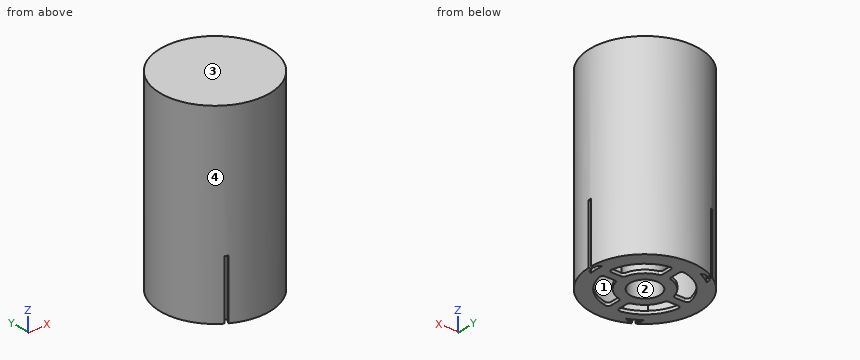
```python
from build123d import *

# Parameters (mm, degrees)
SKETCH_1_R          = 55
EXTRUDE_1_DEPTH     = 190
SKETCH_2_R          = 51.8
CUT_EXTRUDE_1_DEPTH = 186.8
SKETCH_3_R          = 15
CUT_EXTRUDE_2_DEPTH = 10
SKETCH_4_R          = 18.2
SKETCH_4_R_2        = 15
EXTRUDE_2_DEPTH     = 188
SKETCH_5_R          = 55
EXTRUDE_5_DEPTH     = 3.2
EXTRUDE_6_DEPTH     = 1.5
EXTRUDE_START       = -63.2
EXTRUDE_7_DEPTH     = 63.2
CUT_EXTRUDE_START   = -60
CUT_EXTRUDE_4_DEPTH = 60
SKETCH_12_R         = 138.367390037
SKETCH_12_R_2       = 55
CUT_EXTRUDE_5_DEPTH = 135
CUT_EXTRUDE_6_DEPTH = 10


with BuildPart() as part:
    # 草图1 → 凸台-拉伸1 (new body)
    with BuildSketch(Plane.XY):
        Circle(SKETCH_1_R)
    extrude(amount=EXTRUDE_1_DEPTH)

    # 草图2 → 切除-拉伸1 (cut)
    with BuildSketch(Plane.XY.offset(190)):
        Circle(SKETCH_2_R)
    extrude(amount=-CUT_EXTRUDE_1_DEPTH, mode=Mode.SUBTRACT)

    # 草图3 → 切除-拉伸2 (cut)
    with BuildSketch(Plane(origin=(0, 0, 0), x_dir=(-1, 0, 0), z_dir=(0, 0, -1))):
        Circle(SKETCH_3_R)
    extrude(amount=-CUT_EXTRUDE_2_DEPTH, mode=Mode.SUBTRACT)

    # 草图4 → 凸台-拉伸2 (add)
    with BuildSketch(Plane.XY.offset(3.2)):
        Circle(SKETCH_4_R)
        with Locations(Location((0, 0, 0), (0, 0, 180))):
            Circle(SKETCH_4_R_2, mode=Mode.SUBTRACT)
    extrude(amount=EXTRUDE_2_DEPTH)

    # 草图5 → 凸台-拉伸5 (add)
    with BuildSketch(Plane.XY.offset(190)):
        Circle(SKETCH_5_R)
    extrude(amount=EXTRUDE_5_DEPTH)

    # 草图8 → 凸台-拉伸6 (add, symmetric)
    with BuildSketch(Plane(origin=(0, 0, 0), x_dir=(-1, 0, 0), z_dir=(0, 1, 0))):
        Polygon((-55, 90), (-135, 65), (-135, -15), (-55, 0), (-53, 0), (-53, 90), align=None)
    extrude(amount=EXTRUDE_6_DEPTH, both=True)

    # 草图9 → 凸台-拉伸7 (add)
    with BuildSketch(Plane(origin=(0, 0, 0), x_dir=(-1, 0, 0), z_dir=(0, 0, -1)).offset(EXTRUDE_START)):
        with BuildLine():
            Line((-51.178511116, 8), (-47.866376508, 9.5))
            Line((-47.866376508, 9.5), (-44.599439458, 9.5))
            ThreePointArc((-44.599439458, 9.5), (-45.6, 0), (-44.599439458, -9.5))
            Line((-44.599439458, -9.5), (-47.866376508, -9.5))
            Line((-47.866376508, -9.5), (-51.178511116, -8))
            ThreePointArc((-51.178511116, -8), (-51.8, 0), (-51.178511116, 8))
        make_face()
        with BuildLine():
            Line((32.517458788, 40.321890754), (32.16042959, 36.703498043))
            Line((32.16042959, 36.703498043), (30.526961065, 33.874247565))
            ThreePointArc((30.526961065, 33.874247565), (22.8, 39.490758413), (14.072478393, 43.374247565))
            Line((14.072478393, 43.374247565), (15.705946918, 46.203498043))
            Line((15.705946918, 46.203498043), (18.661052327, 48.321890754))
            ThreePointArc((18.661052327, 48.321890754), (25.9, 44.860115916), (32.517458788, 40.321890754))
        make_face()
        with BuildLine():
            Line((18.661052327, -48.321890754), (15.705946918, -46.203498043))
            Line((15.705946918, -46.203498043), (14.072478393, -43.374247565))
            ThreePointArc((14.072478393, -43.374247565), (22.8, -39.490758413), (30.526961065, -33.874247565))
            Line((30.526961065, -33.874247565), (32.16042959, -36.703498043))
            Line((32.16042959, -36.703498043), (32.517458788, -40.321890754))
            ThreePointArc((32.517458788, -40.321890754), (25.9, -44.860115916), (18.661052327, -48.321890754))
        make_face()
    extrude(amount=EXTRUDE_7_DEPTH)

    # 草图11 → 切除-拉伸4 (cut)
    with BuildSketch(Plane(origin=(0, 0, 0), x_dir=(-1, 0, 0), z_dir=(0, 0, -1)).offset(CUT_EXTRUDE_START)):
        with BuildLine():
            Line((-65.998357279, 1.5), (-51.778277298, 1.5))
            ThreePointArc((-51.778277298, 1.5), (-51.697827643, 3.251863624), (-51.558122541, 5))
            Line((-51.558122541, 5), (-48.29534139, 7))
            ThreePointArc((-48.29534139, 7), (-48.8, 0), (-48.29534139, -7))
            Line((-48.29534139, -7), (-51.558122541, -5))
            ThreePointArc((-51.558122541, -5), (-51.697827643, -3.251863624), (-51.778277298, -1.5))
            Line((-51.778277298, -1.5), (-65.998357279, -1.5))
            Line((-65.998357279, -1.5), (-65.998357279, 1.5))
        make_face()
        with BuildLine():
            Line((34.298216745, 56.406254012), (31.700140534, 57.906254012))
            Line((31.700140534, 57.906254012), (24.590100544, 45.591303505))
            ThreePointArc((24.590100544, 45.591303505), (23.032717313, 46.397563871), (21.448934252, 47.150643892))
            Line((21.448934252, 47.150643892), (18.085492869, 45.324992528))
            ThreePointArc((18.085492869, 45.324992528), (24.4, 42.262039705), (30.209848522, 38.324992528))
            Line((30.209848522, 38.324992528), (30.10918829, 42.150643892))
            ThreePointArc((30.10918829, 42.150643892), (28.665110329, 43.145700247), (27.188176755, 44.091303505))
            Line((27.188176755, 44.091303505), (34.298216745, 56.406254012))
        make_face()
        with BuildLine():
            Line((31.700140534, -57.906254012), (34.298216745, -56.406254012))
            Line((34.298216745, -56.406254012), (27.188176755, -44.091303505))
            ThreePointArc((27.188176755, -44.091303505), (28.665110329, -43.145700247), (30.10918829, -42.150643892))
            Line((30.10918829, -42.150643892), (30.209848522, -38.324992528))
            ThreePointArc((30.209848522, -38.324992528), (24.4, -42.262039705), (18.085492869, -45.324992528))
            Line((18.085492869, -45.324992528), (21.448934252, -47.150643892))
            ThreePointArc((21.448934252, -47.150643892), (23.032717313, -46.397563871), (24.590100544, -45.591303505))
            Line((24.590100544, -45.591303505), (31.700140534, -57.906254012))
        make_face()
    extrude(amount=CUT_EXTRUDE_4_DEPTH, mode=Mode.SUBTRACT)

    # 草图12 → 切除-拉伸5 (cut, symmetric)
    with BuildSketch(Plane(origin=(0, 0, 0), x_dir=(-1, 0, 0), z_dir=(0, 0, -1))):
        Circle(SKETCH_12_R)
        with Locations(Location((0, 0, 0), (0, 0, 58.437194054))):
            Circle(SKETCH_12_R_2, mode=Mode.SUBTRACT)
    extrude(amount=CUT_EXTRUDE_5_DEPTH, both=True, mode=Mode.SUBTRACT)

    # 草图13 → 切除-拉伸6 (cut)
    with BuildSketch(Plane(origin=(0, 0, 0), x_dir=(-1, 0, 0), z_dir=(0, 0, -1))):
        with BuildLine():
            Line((4, 27.110883423), (4, 36.331804249))
            ThreePointArc((4, 36.331804249), (5.08985638, 38.645103052), (7.567567568, 39.277626215))
            ThreePointArc((7.567567568, 39.277626215), (28.284271247, 28.284271247), (39.277626215, 7.567567568))
            ThreePointArc((39.277626215, 7.567567568), (38.645103052, 5.08985638), (36.331804249, 4))
            Line((36.331804249, 4), (27.110883423, 4))
            ThreePointArc((27.110883423, 4), (25.273766116, 4.628291755), (24.206145914, 6.25))
            ThreePointArc((24.206145914, 6.25), (17.67766953, 17.67766953), (6.25, 24.206145914))
            ThreePointArc((6.25, 24.206145914), (4.628291755, 25.273766116), (4, 27.110883423))
        make_face()
        with BuildLine():
            Line((-4, 27.110883423), (-4, 36.331804249))
            ThreePointArc((-4, 36.331804249), (-5.08985638, 38.645103052), (-7.567567568, 39.277626215))
            ThreePointArc((-7.567567568, 39.277626215), (-28.284271247, 28.284271247), (-39.277626215, 7.567567568))
            ThreePointArc((-39.277626215, 7.567567568), (-38.645103052, 5.08985638), (-36.331804249, 4))
            Line((-36.331804249, 4), (-27.110883423, 4))
            ThreePointArc((-27.110883423, 4), (-25.273766116, 4.628291755), (-24.206145914, 6.25))
            ThreePointArc((-24.206145914, 6.25), (-17.67766953, 17.67766953), (-6.25, 24.206145914))
            ThreePointArc((-6.25, 24.206145914), (-4.628291755, 25.273766116), (-4, 27.110883423))
        make_face()
        with BuildLine():
            Line((27.110883423, -4), (36.331804249, -4))
            ThreePointArc((36.331804249, -4), (38.645103052, -5.08985638), (39.277626215, -7.567567568))
            ThreePointArc((39.277626215, -7.567567568), (28.284271247, -28.284271247), (7.567567568, -39.277626215))
            ThreePointArc((7.567567568, -39.277626215), (5.08985638, -38.645103052), (4, -36.331804249))
            Line((4, -36.331804249), (4, -27.110883423))
            ThreePointArc((4, -27.110883423), (4.628291755, -25.273766116), (6.25, -24.206145914))
            ThreePointArc((6.25, -24.206145914), (17.67766953, -17.67766953), (24.206145914, -6.25))
            ThreePointArc((24.206145914, -6.25), (25.273766116, -4.628291755), (27.110883423, -4))
        make_face()
        with BuildLine():
            Line((-4, -27.110883423), (-4, -36.331804249))
            ThreePointArc((-4, -36.331804249), (-5.08985638, -38.645103052), (-7.567567568, -39.277626215))
            ThreePointArc((-7.567567568, -39.277626215), (-28.284271247, -28.284271247), (-39.277626215, -7.567567568))
            ThreePointArc((-39.277626215, -7.567567568), (-38.645103052, -5.08985638), (-36.331804249, -4))
            Line((-36.331804249, -4), (-27.110883423, -4))
            ThreePointArc((-27.110883423, -4), (-25.273766116, -4.628291755), (-24.206145914, -6.25))
            ThreePointArc((-24.206145914, -6.25), (-17.67766953, -17.67766953), (-6.25, -24.206145914))
            ThreePointArc((-6.25, -24.206145914), (-4.628291755, -25.273766116), (-4, -27.110883423))
        make_face()
    extrude(amount=-CUT_EXTRUDE_6_DEPTH, mode=Mode.SUBTRACT)


solid = part.part
```
Verification items for the finished model (mm, model axes). Face numbers are marked on the shaded views. Give positions to 0.01 mm unless a question says otherwise; leave off trailing zeros. Loops run counter-clockwise (first coordinate to the right, second up) from the corner with the lowest first, then second, coordinate; pieces in that order, holes last. Notation, with made-up numbers: M 83,81 L 113,81 A30 ccw 113,114 Z; hole C 11.25,69.5 d2. An arc over 180 degrees is marked long. One line per question, with ' | ' between items.
Item 1: Section check D-D, the plane z = 45. State how many separate pieces and enclosed holes the cut face has, plus the area to 3 significant figures.
Completed:
separate pieces: 2 | enclosed holes: 2 | area: 1,610 mm^2
Item 2: Depth check by flat-ended pin: P1, Ø11, axis at x = -21, y = 43.5, coming from the -Z side; P2, Ø24, axis at x = 1, y = 0, coming from the -Z side; P3, Ø3.5, axis at y = -30, z = 1.5, coming from the -X side; P4, Ø3, axis at x = -14, z = 60.5, coming from the -Y side. Enter the tip coordinate at first touch or a pass-through.
Completed:
P1: stops at z = 0 | P2: stops at z = 190 | P3: stops at x = -47.19 | P4: stops at y = -53.56
Item 3: Section check A-A, the plane x = 0. Record the cut outline in (y, z), plus the area to 3 significant figures.
Completed:
outline: M -55,0 L -15,0 L -15,190 L 15,190 L 15,0 L 55,0 L 55,193.2 L -55,193.2 Z; hole M -51.8,3.2 L -18.2,3.2 L -18.2,190 L -51.8,190 Z; hole M 18.2,3.2 L 51.8,3.2 L 51.8,190 L 18.2,190 Z | area: 3,000 mm^2
Item 4: Thickness scan on line 1 (Y direction, x = 0, z = 133.5); line 2 (Z direction, x = 20, y = -9); line 3 (X direction, y = 10, z = 26.5). Record the ranges inside material, lowest first. Write a range as [from, to].
Completed:
line 1: y = [-55, -51.8], [-18.2, -15], [15, 18.2], [51.8, 55] | line 2: z = [0, 3.2], [190, 193.2] | line 3: x = [-54.08, -50.83], [-15.21, -11.18], [11.18, 15.21], [50.83, 54.08]
Item 5: Section check B-B, the plane z = 138. Record the cut outline in (x, y), plus the area to 3 significant figures.
Completed:
outline: C 0,0 d110; C 0,0 d36.4; hole C 0,0 d103.6; hole C 0,0 d30 | area: 1,410 mm^2
Item 6: Draft check along Y on the marked faces 1, 2, 3 and 4. Enter one of: +Y half, -Y half, draft (parallel to the pull), parting line (faces both ways), or undercut.
Completed:
face 1: undercut | face 2: undercut | face 3: draft | face 4: parting line
Item 7: Section check C-C, the plane y = 21. Record the cut outline in (x, z).
Completed:
outline: M -50.83,0 L -34.04,0 L -34.04,3.2 L -47.35,3.2 L -47.35,190 L 47.35,190 L 47.35,3.2 L 34.04,3.2 L 34.04,0 L 50.83,0 L 50.83,193.2 L -50.83,193.2 Z; M -13.56,0 L 13.56,0 L 13.56,3.2 L -13.56,3.2 Z
